Autodesk Inventor part; units mm, degrees
ref_plane "Work Plane1" through (0, 0, -70) normal (0, 0, 1) x (1, 0, 0)
ref_plane "Work Plane2" through (0, -50, 0) normal (0, 1, 0) x (-1, 0, 0)
ref_plane "Work Plane3" through (-310, 0, 0) normal (1, 0, 0) x (0, 1, 0)
ref_plane "Work Plane1" through (0, 0, -70) normal (0, 0, 1) x (1, 0, 0)
ref_plane "Work Plane2" through (0, -50, 0) normal (0, 1, 0) x (-1, 0, 0)
ref_plane "Work Plane3" through (-310, 0, 0) normal (1, 0, 0) x (0, 1, 0)
sketch "Sketch2" plane through (0, 0, -70) normal (0, 0, 1) x (1, 0, 0)
  line L0 (0, 0) -> (-60, -50) construction
  line L1 (-60, -50) -> (-310, -50) construction
  line L2 (-310, 10) -> (-310, -60) construction
  dimension "d3" = 250
  dimension "d4" = 50
sketch "Sketch3" plane through (-310, 0, 0) normal (1, 0, 0) x (0, 1, 0)
  line L0 (-50, -70) -> (-50, -15) construction
  line L1 (-50, -15) -> (-17.5, -15) construction
  dimension "d5" = 55
  dimension "d6" = 32.5
ref_plane "Work Plane4" through (-310, -17.5, -15) normal (0, 1, 0) x (-1, 0, 0)
sketch "Sketch4" plane through (-310, -17.5, -15) normal (0, 1, 0) x (-1, 0, 0)
  line L0 (0, 0) -> (-25, 0) construction
  dimension "d7" = 25
sketch "Sketch5" plane through (0, 0, 0) normal (0, 0, 1) x (1, 0, 0)
  circle A0 centre (0, 0) radius 2.5
  dimension "d13" = 5
sketch3d "3D Sketch1"
  line L0 (0, 0, 0) -> (0, 0, -60)
  arc A0 (0, 0, -60) -> (-7.6822, -6.4018, -70) centre (-7.6822, -6.4018, -60) ccw
  line L1 (-7.6822, -6.4018, -70) -> (-46.0933, -38.4111, -70)
  arc A1 (-46.0933, -38.4111, -70) -> (-78.1025, -50, -70) centre (-78.1025, 0, -70) ccw
  line L2 (-78.1025, -50, -70) -> (-300, -50, -70)
  arc A2 (-300, -50, -70) -> (-310, -50, -60) centre (-300, -50, -60) ccw
  line L3 (-310, -50, -60) -> (-310, -50, -25)
  arc A3 (-310, -50, -25) -> (-310, -40, -15) centre (-310, -40, -25) ccw
  line L4 (-310, -40, -15) -> (-310, -27.5, -15)
  arc A4 (-310, -27.5, -15) -> (-300, -17.5, -15) centre (-300, -27.5, -15) ccw
  line L5 (-300, -17.5, -15) -> (-285, -17.5, -15)
  dimension "d8" = 10
  dimension "d9" = 10
  dimension "d10" = 10
  dimension "d11" = 10
  dimension "d12" = 50
sweep "Sweep1" add profiles "Sketch5" path "3D Sketch1"
equation "\"d9\" = d8"
equation "\"d10\" = d8"
equation "\"d11\" = d8"
properties part number "314-15" material "Steel"
Verification items for the finished model (mm, model axes). A direction names the side the tool comes from. Give positions to 0.01 mm unless a question says otherwise; leave off trailing zeros. Return JSON: item names as keys, results as strings. Group by question number.
1) Scan lines: line 1 (X direction, y = -2, z = -37); line 2 (Z direction, x = -71.5, y = -48.5); line 3 (X direction, y = -49, z = -34.5). Record each from-to range of solid material in increasing order.
2) Access from +Z, -Z, +X, -X, +Y, -Y to the whole of each face (thin tool, end or side, straight path). Record for faces 1 (the face through (-0.54, 2.44, -30.42)), 2 (the face through (0, 0, 0)).
3) Go/stop test with flat-tipped pins: pin 1 Ø5 at (x, y) = (-267.5, -46.5) entering from -Z; pin 2 Ø1.5 at (y, z) = (-16.5, -14.5) entering from +X; pin 3 Ø12 at (y, z) = (-6.5, -33) entering from -X. Record where each tip stops, or that it passes through.
Answer block:
{
 "1": {"line 1": "x = -1.5 to 1.5", "line 2": "z = -72.27 to -67.73", "line 3": "x = -312.29 to -307.71"},
 "2": {"face 1": "+Z", "face 2": "+Z, +X, -X, +Y, -Y"},
 "3": {"pin 1": "stops at z = -72.29", "pin 2": "stops at x = -285", "pin 3": "stops at x = -2.45"}
}
